Here's how the part is built. I have some questions about the finished solid (model axes, mm). A direction names the side the tool comes from. Give positions to 0.01 mm unless a question says otherwise; leave off trailing zeros. Loops run counter-clockwise (first coordinate to the right, second up) from the corner with the lowest first, then second, coordinate; pieces in that order, holes last. Notation, with made-up numbers: (85, 62.25) - (119, 62.25) arc R27 ccw to (119, 89.25) - close; hole circle Ø10 at (13.5, 52). An arc over 180 degrees is marked (long way). Put each result on its own line as item: value. Start each with the question number.
from build123d import *

# Parameters (mm, degrees)
SKETCH_1_R               = 1.5
EXTRUDE_1_DEPTH          = 15
CUT_EXTRUDE_2_DEPTH      = 79.576395947
CUT_EXTRUDE_2_DEPTH_BACK = 79.576395947
SKETCH_2_W               = 6
SKETCH_2_H               = 12
CUT_EXTRUDE_3_DEPTH      = 83.692200358
CUT_EXTRUDE_3_DEPTH_BACK = 83.692200358
SKETCH_3_W               = 0.5
SKETCH_3_H               = 10
CUT_EXTRUDE_4_DEPTH      = 79.576395947
CUT_EXTRUDE_4_DEPTH_BACK = 79.576395947
SKETCH_4_R               = 5.25


with BuildPart() as part:
    # 草图1 → 凸台-拉伸1 (new, symmetric)
    with BuildSketch(Plane.XY):
        with BuildLine():
            Line((0, -3), (77, -3))
            Line((77, -3), (77, -1.5))
            Line((77, -1.5), (3.354101966, -1.5))
            ThreePointArc((3.354101966, -1.5), (2.953210103, -1.298807152), (2.874944542, -0.857142857))
            ThreePointArc((2.874944542, -0.857142857), (-1.792842914, 2.405351177), (0, -3))
        make_face()
        Circle(SKETCH_1_R, mode=Mode.SUBTRACT)
    extrude(amount=EXTRUDE_1_DEPTH, both=True)

    # 草图2 → 切除-拉伸2 (cut, two sides: drawn at the far end of the back side and taken through both)
    with BuildSketch(Plane(origin=(0, -1.5, 0), x_dir=(1, 0, 0), z_dir=(0, 1, 0)).offset(-CUT_EXTRUDE_2_DEPTH_BACK)):
        Rectangle(SKETCH_2_W, SKETCH_2_H)
    extrude(amount=CUT_EXTRUDE_2_DEPTH + CUT_EXTRUDE_2_DEPTH_BACK, mode=Mode.SUBTRACT)

    # 草图3 → 切除-拉伸3 (cut, two sides: drawn at the far end of the back side and taken through both)
    with BuildSketch(Plane.XY.offset(15).offset(-CUT_EXTRUDE_3_DEPTH_BACK)):
        with Locations((-0.25, -5)):
            Rectangle(SKETCH_3_W, SKETCH_3_H)
    extrude(amount=CUT_EXTRUDE_3_DEPTH + CUT_EXTRUDE_3_DEPTH_BACK, mode=Mode.SUBTRACT)

    # 草图4 → 切除-拉伸4 (cut, two sides: drawn at the far end of the back side and taken through both)
    with BuildSketch(Plane(origin=(0, -1.5, 0), x_dir=(1, 0, 0), z_dir=(0, 1, 0)).offset(-CUT_EXTRUDE_4_DEPTH_BACK)):
        with Locations(Location((19, 0, 0), (0, 0, 270))):
            Circle(SKETCH_4_R)
        with Locations(Location((49, 0, 0), (0, 0, 270))):
            Circle(SKETCH_4_R)
    extrude(amount=CUT_EXTRUDE_4_DEPTH + CUT_EXTRUDE_4_DEPTH_BACK, mode=Mode.SUBTRACT)


solid = part.part
1) Suppose I cut it at C-C on z = 0. Please give me the cut outline in (x, y).
2) I need wall thicknesses on line 1 (X direction, y = 0, z = -8); line 2 (Z direction, x = 49, y = -2.55); line 3 (Y direction, x = 21, z = 5.75). Which ranges of each line are inside material? Lowest first, please.
3) Thinking about a two-plate mould opening in X: for faces 1 (the flat face through (77, -2, 0)), 2 (the flat face through (1.3, -1.4, 6)), 3 (the flat face through (-0.5, -2, 10)), 4 (the cylindrical face through (0.315, 1.467, -10.563)), which applies, pulls with the +X half, pulls with the -X half, needs draft (parallel to the pull), parting line crosses it, or undercut?
4) Suppose I cut it at D-D on x = 17.5. Please give me the cut outline in (y, z), plus the area to 3 significant figures.
5) Suppose I cut it at B-B on x = 49. Please give me the cut outline in (y, z).
6) I'm going to push flat-ended pins straight in: P1, Ø3, axis at y = -2, z = 9, coming from the -X side; P2, Ø5, axis at x = 35.5, z = -9.5, coming from the +Y side; P3, Ø0.8, axis at y = -2, z = -9.5, coming from the -X side. Where does each tip first touch, or does it pass through?
7) Suppose I cut it at A-A on y = 0. Please give me the cut outline in (x, z), plus the area to 3 significant figures.
8) Which directions (+Z, -Z, +X, -X, +Y, -Y) give clear straight access to the entire face, cutting with the end or side of a thin tool? Please do faces 5 (the flat face through (1.3, -1.4, -6)), 6 (the flat face through (41, -1.5, 0)), 7 (the flat face through (-0.5, -2, -11)).
Ans:
1. outline: (3, -3) - (13.75, -3) - (13.75, -1.5) - (3.35, -1.5) arc R0.5 cw to (3, -1.35) - close; (24.25, -3) - (43.75, -3) - (43.75, -1.5) - (24.25, -1.5) - close; (54.25, -3) - (77, -3) - (77, -1.5) - (54.25, -1.5) - close
2. line 1: x = -3 to -1.5, 1.5 to 3
2. line 2: z = -15 to -5.25, 5.25 to 15
2. line 3: y = -3 to -1.5
3. face 1: pulls with the +X half
3. face 2: needs draft
3. face 3: undercut
3. face 4: undercut
4. outline: (-3, -15) - (-1.5, -15) - (-1.5, -5.03) - (-3, -5.03) - close; (-3, 5.03) - (-1.5, 5.03) - (-1.5, 15) - (-3, 15) - close
4. area: 29.9 mm²
5. outline: (-3, -15) - (-1.5, -15) - (-1.5, -5.25) - (-3, -5.25) - close; (-3, 5.25) - (-1.5, 5.25) - (-1.5, 15) - (-3, 15) - close
6. P1: stops at x = -2.96
6. P2: stops at y = -1.5
6. P3: stops at x = -2.54
7. outline: (-3, -15) - (-1.5, -15) - (-1.5, -6) - (-3, -6) - close; (-3, 6) - (-1.5, 6) - (-1.5, 15) - (-3, 15) - close; (1.5, -15) - (3, -15) - (3, -6) - (1.5, -6) - close; (1.5, 6) - (3, 6) - (3, 15) - (1.5, 15) - close
7. area: 54.0 mm²
8. face 5: -X, +Y, -Y
8. face 6: +Z, -Z, +X, +Y
8. face 7: +Z, -Z, -Y
